Verification items for the finished model (mm, model axes). A direction names the side the tool comes from. Round coordinates to 2 decimals unless told otherwise and drop trailing zeros. Write each loop counter-clockwise with the first axis right and the second up, starting at its lowest first coordinate (ties: lowest second). Pieces come first, ordered by that corner, then holes. Notation, with made-up numbers: (49.25, 60.5) - (73.25, 60.5) arc R11 cw to (73.25, 73.5) - close; hole circle Ø11 at (53.25, 73.25). An arc over 180 degrees is marked (long way). Answer as a JSON object with one key per item and string values.
```python
from build123d import *

# Parameters (mm, degrees)
F0_W         = 35
F0_H         = 30
F0_R         = 1.25
F1_DEPTH     = 2
F2_W         = 20
F2_H         = 20
F2_W_2       = 30
F2_W_3       = 10
F3_DEPTH     = 4
F4_T4_DEPTH  = 2
F4_T9_DEPTH  = 2
F4_T14_DEPTH = 2
F4_T19_DEPTH = 2
F6_SIZE      = 5.08
F7_SIZE      = 5.08
F9_DEPTH     = 2
F10_T1_DEPTH = 20


# Not quite as in the source:
# - a fillet or chamfer that OpenCascade refuses, or shapes differently, is made with other operations: its cross-section is extruded or revolved along the edge and cut away or added
# - a feature of the source that left no trace in its solid (it failed there, or was rolled back) is left out


with BuildPart() as f1:
    # F0 (on Top) → F1 (new body)
    with BuildSketch(Plane.XY):
        Rectangle(F0_W, F0_H)
        with Locations((-14.45, -11.95)):
            Circle(F0_R, mode=Mode.SUBTRACT)
        Polygon((-8.9161582291, 8.9178942144), (8.9161582291, 8.9178942144), (10.7079278678, 8.9178942144), (10.7079250291, -8.9178942144), (8.9161582291, -8.9178942144), (-8.9161582291, -8.9178942144), (-8.9161582291, -6.7814155482), (-13.8649037108, -6.7814155482), (-13.8649037108, 6.1875791289), (-8.9161582291, 6.1875791289), align=None, mode=Mode.SUBTRACT)
        with Locations((-14.45, 11.95)):
            Circle(F0_R, mode=Mode.SUBTRACT)
        with Locations((14.45, 0)):
            Circle(F0_R, mode=Mode.SUBTRACT)
    extrude(amount=F1_DEPTH)

    # F2 (on face) → F3 (join)
    with BuildSketch(Plane.XY.offset(2)):
        with BuildLine():
            Line((47.5, 10), (47.5, -10))
            ThreePointArc((47.5, -10), (54.6755987692, 0), (47.5, 10))
        make_face()
        with BuildLine():
            ThreePointArc((-47.5, 10), (-54.6755833881, 0), (-47.5, -10))
            Line((-47.5, -10), (-47.5, 10))
        make_face()
        with Locations((37.5, 0)):
            Rectangle(F2_W, F2_H)
        with Locations((-32.5, 0)):
            Rectangle(F2_W_2, F2_H)
        with Locations((22.5, 0)):
            Rectangle(F2_W_3, F2_H)
    extrude(amount=-F3_DEPTH)

    # F4: chamfer of 5.08 on 4 edges, made by hand


with BuildPart() as f4_tool2:
    # F4_s3 → F4_t4 (new body)
    with BuildSketch(Plane.XY.offset(2)):
        Polygon((-17.5, 15.08), (-22.58, 10), (-17.5, 10), align=None)
    extrude(amount=-F4_T4_DEPTH)

    split(bisect_by=Plane.XZ.offset(-15), keep=Keep.TOP)


with BuildPart() as f1_1:
    add(f1.part)

    # F4_t1: union F4_tool2
    add(f4_tool2.part)


with BuildPart() as f4_tool7:
    # F4_s8 → F4_t9 (new body)
    with BuildSketch(Plane.XY.offset(2)):
        Polygon((17.5, -15.08), (22.58, -10), (17.5, -10), align=None)
    extrude(amount=-F4_T9_DEPTH)

    split(bisect_by=Plane.XZ.offset(15), keep=Keep.BOTTOM)


with BuildPart() as f1_2:
    add(f1_1.part)

    # F4_t6: union F4_tool7
    add(f4_tool7.part)


with BuildPart() as f4_tool12:
    # F4_s13 → F4_t14 (new body)
    with BuildSketch(Plane.XY.offset(2)):
        Polygon((17.5, 15.08), (22.58, 10), (17.5, 10), align=None)
    extrude(amount=-F4_T14_DEPTH)

    split(bisect_by=Plane.XZ.offset(-15), keep=Keep.TOP)


with BuildPart() as f1_3:
    add(f1_2.part)

    # F4_t11: union F4_tool12
    add(f4_tool12.part)


with BuildPart() as f4_tool17:
    # F4_s18 → F4_t19 (new body)
    with BuildSketch(Plane.XY.offset(2)):
        Polygon((-17.5, -15.08), (-22.58, -10), (-17.5, -10), align=None)
    extrude(amount=-F4_T19_DEPTH)

    split(bisect_by=Plane.XZ.offset(15), keep=Keep.BOTTOM)


with BuildPart() as f1_4:
    add(f1_3.part)

    # F4_t16: union F4_tool17
    add(f4_tool17.part)

    # F6
    f6_edges = [f1_4.edges().sort_by_distance(p)[0] for p in [
        (17.5, -10, -1),
    ]]
    chamfer(f6_edges, length=F6_SIZE)

    # F7
    f7_edges = [f1_4.edges().sort_by_distance(p)[0] for p in [
        (17.5, 10, -1),
    ]]
    chamfer(f7_edges, length=F7_SIZE)

    # F8 (on face) → F9 (cut)
    with BuildSketch(Plane(origin=(0, 0, -2), x_dir=(1, 0, 0), z_dir=(0, 0, -1))):
        Polygon((27.5, -10), (27.5, 10), (22.58, 10), (17.5, 4.92), (17.5, -4.92), (22.58, -10), align=None)
    extrude(amount=-F9_DEPTH, mode=Mode.SUBTRACT)

    # F10: fillet of radius 5.08 on 1 edges, made by hand

    # F10_s2 → F10_t1 (join)
    with BuildSketch(Plane.XZ.offset(-10)):
        with BuildLine():
            ThreePointArc((27.5, -2), (25.7140835586, -0.5273743839), (23.4601980247, 0))
            Line((23.4601980247, 0), (27.5, 0))
            Line((27.5, 0), (27.5, -2))
        make_face()
    extrude(amount=F10_T1_DEPTH)


solid = f1_4.part
```
1. Go/stop test with flat-tipped pins: pin 1 (2 mm diameter, centred on y = -8, z = 1, fed in from +X); pin 2 (3 mm diameter, centred on x = 14.45, y = 0, fed in from -Z); pin 3 (1 mm diameter, centred on y = 1.5, z = 1, fed in from +X). Record where each tip stops, or that it passes through.
Completed:
{"pin 1": "stops at x = 52.02", "pin 2": "stops at z = 0", "pin 3": "stops at x = 54.63"}
2. Cross-section at C-C (y = 0). Record the boundary of the cut face in (x, z).
Completed:
{"outline": "(-54.68, -2) - (-17.5, -2) - (-17.5, 0) - (-13.86, 0) - (-13.86, 2) - (-54.68, 2) - close; (10.71, 0) - (13.2, 0) - (13.2, 2) - (10.71, 2) - close; (15.7, 0) - (23.46, 0) arc R5.08 cw to (27.5, -2) - (54.68, -2) - (54.68, 2) - (15.7, 2) - close"}
3. Cross-section at D-D (z = 0.95). Record the boundary of the cut face in (x, y), plus the area to 3 significant figures.
Completed:
{"outline": "(-47.5, -10) - (-22.58, -10) - (-17.58, -15) - (17.58, -15) - (22.58, -10) - (47.5, -10) arc R10.56 ccw to (47.5, 10) - (22.58, 10) - (17.58, 15) - (-17.58, 15) - (-22.58, 10) - (-47.5, 10) arc R10.56 ccw to start; hole circle Ø2.5 at (-14.45, -11.95); hole circle Ø2.5 at (-14.45, 11.95); hole (-13.86, -6.78) - (-8.92, -6.78) - (-8.92, -8.92) - (10.71, -8.92) - (10.71, 8.92) - (-8.92, 8.92) - (-8.92, 6.19) - (-13.86, 6.19) - close; hole circle Ø2.5 at (14.45, 0)", "area": "2,080 mm^2"}
4. Cross-section at B-B (x = 14.45). Record the boundary of the cut face in (y, z), plus the area to 3 significant figures.
Completed:
{"outline": "(-15, 0) - (-1.25, 0) - (-1.25, 2) - (-15, 2) - close; (1.25, 0) - (15, 0) - (15, 2) - (1.25, 2) - close", "area": "55.0 mm^2"}
5. Material ranges on probe 1 along Y at (x, z) = (-14.45, 1.5); probe 2 along Y at (x, z) = (-12, 1.35); probe 3 along Y at (x, z) = (14.45, 1.15), recorded low to high. Write a range as from..to.
Completed:
{"probe 1": "y = -15..-13.2, -10.7..10.7, 13.2..15", "probe 2": "y = -15..-6.78, 6.19..15", "probe 3": "y = -15..-1.25, 1.25..15"}
6. Cross-section at A-A (y = -11.95). Record the boundary of the cut face in (x, z), plus the area to 3 significant figures.
Completed:
{"outline": "(-20.63, 0) - (-15.7, 0) - (-15.7, 2) - (-20.63, 2) - close; (-13.2, 0) - (20.63, 0) - (20.63, 2) - (-13.2, 2) - close", "area": "77.5 mm^2"}
7. Access from +Z, -Z, +X, -X, +Y, -Y to the whole of each face (thin tool, end or side, straight path). Record for faces 5 (the face through (-17.5, 0, -1)), 6 (the face through (0, 15, 1)), 7 (the face through (1, 8.918, 1)).
Completed:
{"face 5": "-Z, +Y, -Y", "face 6": "+Z, -Z, +X, -X, +Y", "face 7": "+Z, -Z"}
8. Mould release check, pull along X, two halves, no side actions. Record for faces 1 (the face through (-13.865, 0, 1)), 2 (the face through (1, -10, 2)), 3 (the face through (-54.674, 0.184, 0.028)), 4 (the face through (20.04, -12.54, 1.01)): released by +X, released by -X, zero draft, split by the parting line, or undercut.
Completed:
{"face 1": "undercut", "face 2": "zero draft", "face 3": "released by -X", "face 4": "released by +X"}
